Autodesk Inventor part; units mm, degrees
ref_plane "YZ Plane" through (0, 0, 0) normal (1, 0, 0) x (0, 1, 0)
ref_plane "XZ Plane" through (0, 0, 0) normal (0, 1, 0) x (-1, 0, 0)
ref_plane "XY Plane" through (0, 0, 0) normal (0, 0, 1) x (1, 0, 0)
sketch "Sketch1" plane through (0, 0, 0) normal (0, 1, 0) x (-1, 0, 0)
  line L0 (-229.8634, 7.9265) -> (-229.8634, -272.0735)
  line L1 (0, -264.1469) -> (0, 0)
  line L2 (-114.9317, 7.8456) -> (-114.9317, -271.9925) construction
  line L3 (-229.8634, -132.0735) -> (0, -132.0735) construction
  line L4 (0, -222.0735) -> (-229.8634, -222.0735) construction
  line L5 (0.0192, -20.1711) -> (0, -20.138) construction
  line L6 (0.9366, -42.0735) -> (-229.8634, -42.0735) construction
  line L7 (-39.8418, -42.0735) -> (-39.8418, -2.1597) construction
  line L8 (-39.8418, -5.776) -> (-30, -5.776)
  line L9 (-39.8418, -5.776) -> (-60, -5.776)
  line L10 (-30, -5.776) -> (-60, -5.776) construction
  line L11 (-30, -3.776) -> (-60, -3.776)
  line L12 (-60, -7.776) -> (-30, -7.776)
  arc A0 (-30, -7.776) -> (-30, -3.776) centre (-30, -5.776) ccw
  arc A1 (-60, -3.776) -> (-60, -7.776) centre (-60, -5.776) ccw
  line L13 (-39.8418, -78.371) -> (-30, -78.371)
  line L14 (-39.8418, -78.371) -> (-60, -78.371)
  line L15 (-30, -78.371) -> (-60, -78.371) construction
  line L16 (-30, -80.371) -> (-60, -80.371)
  line L17 (-60, -76.371) -> (-30, -76.371)
  arc A2 (-30, -80.371) -> (-30, -76.371) centre (-30, -78.371) ccw
  arc A3 (-60, -76.371) -> (-60, -80.371) centre (-60, -78.371) ccw
  line L18 (-231.5784, -23.0949) -> (-148.4647, -23.0949) construction
  line L19 (-148.4647, -23.0949) -> (-148.4647, -61.0949) construction
  line L20 (-148.4647, -61.0949) -> (-231.5784, -61.0949) construction
  line L21 (-190.0216, -5.776) -> (-199.8634, -5.776)
  line L22 (-190.0216, -5.776) -> (-169.8634, -5.776)
  line L23 (-199.8634, -5.776) -> (-169.8634, -5.776) construction
  line L24 (-199.8634, -3.776) -> (-169.8634, -3.776)
  line L25 (-169.8634, -7.776) -> (-199.8634, -7.776)
  arc A4 (-199.8634, -3.776) -> (-199.8634, -7.776) centre (-199.8634, -5.776) ccw
  arc A5 (-169.8634, -7.776) -> (-169.8634, -3.776) centre (-169.8634, -5.776) ccw
  arc A6 (-169.8634, -80.371) -> (-169.8634, -76.371) centre (-169.8634, -78.371) ccw
  line L26 (-190.0216, -78.371) -> (-169.8634, -78.371)
  line L27 (-169.8634, -76.371) -> (-199.8634, -76.371)
  line L28 (-190.0216, -78.371) -> (-199.8634, -78.371)
  line L29 (-199.8634, -78.371) -> (-169.8634, -78.371) construction
  line L30 (-199.8634, -80.371) -> (-169.8634, -80.371)
  arc A7 (-199.8634, -76.371) -> (-199.8634, -80.371) centre (-199.8634, -78.371) ccw
  line L31 (-114.9317, -271.9925) -> (-114.9317, 7.8456) construction
  line L32 (0, -222.0735) -> (-229.8634, -222.0735) construction
  line L33 (-15.354, -241.052) -> (-98.4678, -241.052) construction
  line L34 (-98.4678, -241.052) -> (-98.4678, -203.052) construction
  line L35 (-98.4678, -203.052) -> (-15.354, -203.052) construction
  line L36 (-39.8418, -222.0735) -> (-39.8418, -261.9872) construction
  line L37 (-39.8418, -258.371) -> (-30, -258.371)
  line L38 (-39.8418, -258.371) -> (-60, -258.371)
  line L39 (-30, -258.371) -> (-60, -258.371) construction
  line L40 (-30, -260.371) -> (-60, -260.371)
  line L41 (-60, -256.371) -> (-30, -256.371)
  arc A8 (-30, -260.371) -> (-30, -256.371) centre (-30, -258.371) ccw
  arc A9 (-60, -256.371) -> (-60, -260.371) centre (-60, -258.371) ccw
  arc A10 (-60, -183.776) -> (-60, -187.776) centre (-60, -185.776) ccw
  line L42 (-39.8418, -185.776) -> (-60, -185.776)
  line L43 (-60, -187.776) -> (-30, -187.776)
  line L44 (-39.8418, -185.776) -> (-30, -185.776)
  line L45 (-30, -185.776) -> (-60, -185.776) construction
  line L46 (-30, -183.776) -> (-60, -183.776)
  arc A11 (-30, -187.776) -> (-30, -183.776) centre (-30, -185.776) ccw
  line L47 (-148.4647, -241.052) -> (-148.4647, -203.052) construction
  line L48 (-169.8634, -256.371) -> (-199.8634, -256.371)
  line L49 (-190.0216, -258.371) -> (-199.8634, -258.371)
  line L50 (-190.0216, -258.371) -> (-169.8634, -258.371)
  arc A12 (-199.8634, -256.371) -> (-199.8634, -260.371) centre (-199.8634, -258.371) ccw
  line L51 (-199.8634, -260.371) -> (-169.8634, -260.371)
  arc A13 (-169.8634, -260.371) -> (-169.8634, -256.371) centre (-169.8634, -258.371) ccw
  line L52 (-199.8634, -258.371) -> (-169.8634, -258.371) construction
  line L53 (-169.8634, -187.776) -> (-199.8634, -187.776)
  line L54 (-190.0216, -185.776) -> (-199.8634, -185.776)
  arc A14 (-199.8634, -183.776) -> (-199.8634, -187.776) centre (-199.8634, -185.776) ccw
  line L55 (-199.8634, -185.776) -> (-169.8634, -185.776) construction
  line L56 (-199.8634, -183.776) -> (-169.8634, -183.776)
  line L57 (-190.0216, -185.776) -> (-169.8634, -185.776)
  arc A15 (-169.8634, -187.776) -> (-169.8634, -183.776) centre (-169.8634, -185.776) ccw
  line L58 (-148.4647, -203.052) -> (-231.5784, -203.052) construction
  line L59 (-231.5784, -241.052) -> (-148.4647, -241.052) construction
  line L60 (-192.7799, 9.4375) -> (-30.2751, 9.4375)
  line L61 (-192.7799, -273.5844) -> (-30.2751, -273.5844)
  line L62 (-80, -5) -> (-150, -5)
  line L63 (-150, -5) -> (-150, 5)
  line L64 (-150, 5) -> (-80, 5)
  line L65 (-80, 5) -> (-80, -5)
  line L66 (-80, -259.1469) -> (-150, -259.1469)
  line L67 (-150, -259.1469) -> (-150, -269.1469)
  line L68 (-150, -269.1469) -> (-80, -269.1469)
  line L69 (-80, -269.1469) -> (-80, -259.1469)
  line L70 (0, 0) -> (0, 9.4375)
  line L71 (0, 9.4375) -> (-30.2751, 9.4375)
  line L72 (-192.7799, 9.4375) -> (-229.8634, 9.4375)
  line L73 (-229.8634, 9.4375) -> (-229.8634, 7.9265)
  line L74 (0, -264.1469) -> (0, -273.5844)
  line L75 (0, -273.5844) -> (-30.2751, -273.5844)
  line L76 (-192.7799, -273.5844) -> (-229.8634, -273.5844)
  line L77 (-229.8634, -273.5844) -> (-229.8634, -272.0735)
  point P0 (-39.8418, -23.0949)
  point P1 (-45, -5.776)
  point P2 (-45, -78.371)
  point P3 (-190.0216, -42.0735)
  point P4 (-190.0216, -23.0949)
  point P5 (-184.8634, -5.776)
  point P6 (-184.8634, -78.371)
  point P7 (-39.8418, -241.052)
  point P8 (-45, -258.371)
  point P9 (-45, -185.776)
  point P10 (-190.0216, -222.0735)
  point P11 (-190.0216, -241.052)
  point P12 (-184.8634, -185.776)
  point P13 (-184.8634, -258.371)
  point P14 (-114.9317, 2.9056)
  point P15 (-45, -78.371)
  point P16 (-45, -185.776)
  point P17 (-114.9317, -267.0525)
  point P18 (-184.8634, -185.776)
  point P19 (-45, -258.371)
  point P20 (-229.8634, -272.8289)
  dimension "d25" = 4
  dimension "d34" = 30
  dimension "d36" = 280
  dimension "d47" = 45
  dimension "d49" = 45
  dimension "d50" = 45
  dimension "d51" = 229.8634
extrude "Extrusion1" add sketch "Sketch1" along normal blind 10 contours L73 L72 L60 L71 L70 L1 L74 L75 L61 L76 L77 L0 | A0 L12 A1 L11 | L16 A3 L17 A2 | L24 A5 L25 A4 | L30 A7 L27 A6 | L40 A9 L41 A8 | L46 A11 L43 A10 | A13 L51 A12 L48 | L53 A14 L56 A15 | L62 L63 L64 L65 | L69 L68 L67 L66
extrude "Extrusion2" cut sketch "Sketch1" along normal through all contours A0 L12 A1 L11 | L16 A3 L17 A2 | L24 A5 L25 A4 | L30 A7 L27 A6 | L40 A9 L41 A8 | L46 A11 L43 A10 | A13 L51 A12 L48 | L53 A14 L56 A15
extrude "Extrusion4" add sketch "Sketch1" along normal blind 10 contours L73 L72 L60 L71 L70 L1 L74 L75 L61 L76 L77 L0 | A0 L12 A1 L11 | L16 A3 L17 A2 | L24 A5 L25 A4 | L30 A7 L27 A6 | L40 A9 L41 A8 | L46 A11 L43 A10 | A13 L51 A12 L48 | L53 A14 L56 A15 | L62 L63 L64 L65 | L69 L68 L67 L66
extrude "Extrusion5" cut sketch "Sketch1" along normal blind 10 contours L62 L63 L64 L65 | L69 L68 L67 L66
extrude "Extrusion6" cut sketch "Sketch1" along normal blind 10 contours L24 A5 L25 A4
extrude "Extrusion7" cut sketch "Sketch1" along normal blind 10 contours A0 L12 A1 L11 | L16 A3 L17 A2 | L30 A7 L27 A6 | L40 A9 L41 A8 | L46 A11 L43 A10 | A13 L51 A12 L48 | L53 A14 L56 A15
properties part number "floor" material "Brass, Soft Yellow"
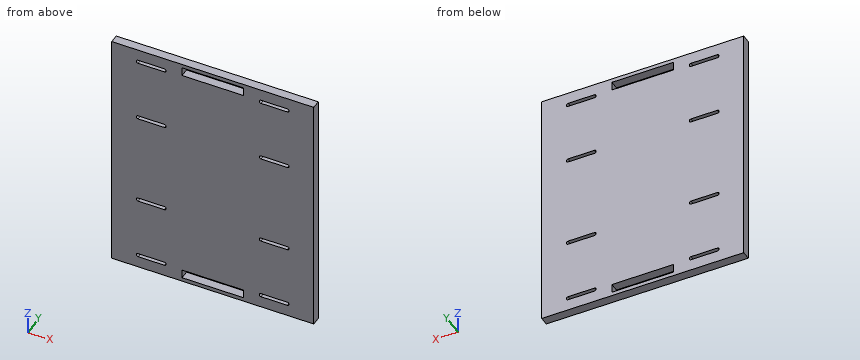
Can you work these out from the model? Positions are in its coordinate system, mm. Round coordinates to 2 decimals unless told otherwise and drop trailing zeros. Loops run counter-clockwise (first coordinate to the right, second up) from the corner with the lowest first, then second, coordinate; pieces in that order, holes last. Notation, with made-up numbers: (-11, -35.75) -> (22, -35.75) arc R23 ccw to (22, -5.75) -> close; hole circle Ø7 at (89, 4.5). An arc over 180 degrees is marked (long way). One line per item, written item: value. Start each with the question number.
1. If we section it at A-A, the plane x = 117: Write out the boundary of the cut face in (y, z), then the cut area to 3 significant figures.
2. If we section it at B-B, the plane x = 36: Write out the boundary of the cut face in (y, z).
3. For pin 1 (5 mm diameter, centred on y = 3, z = -2.5, fed in from -X), with a flat end and sliding along its axis, tell me the tip position at first contact or that it passes through.
4. If I drill on probe 1 along Z at (x, y) = (58.5, 5); probe 2 along Z at (x, y) = (105.5, 1.5); probe 3 along Z at (x, y) = (29.5, 1), over which ranges is the centre line in solid material (lowest first)?
5. If we section it at C-C, the plane y = 8.5: Give the number of separate pieces and of enclosed holes in the cut face, then the cut area to 3 significant figures.
Calculated:
1. outline: (0, -273.58) -> (10, -273.58) -> (10, -269.15) -> (0, -269.15) -> close; (0, -259.15) -> (10, -259.15) -> (10, -5) -> (0, -5) -> close; (0, 5) -> (10, 5) -> (10, 9.44) -> (0, 9.44) -> close
1. area: 2,630 mm²
2. outline: (0, -273.58) -> (10, -273.58) -> (10, -260.37) -> (0, -260.37) -> close; (0, -256.37) -> (10, -256.37) -> (10, -187.78) -> (0, -187.78) -> close; (0, -183.78) -> (10, -183.78) -> (10, -80.37) -> (0, -80.37) -> close; (0, -76.37) -> (10, -76.37) -> (10, -7.78) -> (0, -7.78) -> close; (0, -3.78) -> (10, -3.78) -> (10, 9.44) -> (0, 9.44) -> close
3. pin 1: stops at x = 0
4. probe 1: z = -273.58 to -260.37, -256.37 to -187.78, -183.78 to -80.37, -76.37 to -7.78, -3.78 to 9.44
4. probe 2: z = -273.58 to -269.15, -259.15 to -5, 5 to 9.44
4. probe 3: z = -273.58 to -260.31, -256.43 to -187.71, -183.84 to -80.31, -76.43 to -7.71, -3.84 to 9.44
5. separate pieces: 1
5. enclosed holes: 10
5. area: 62,600 mm²
